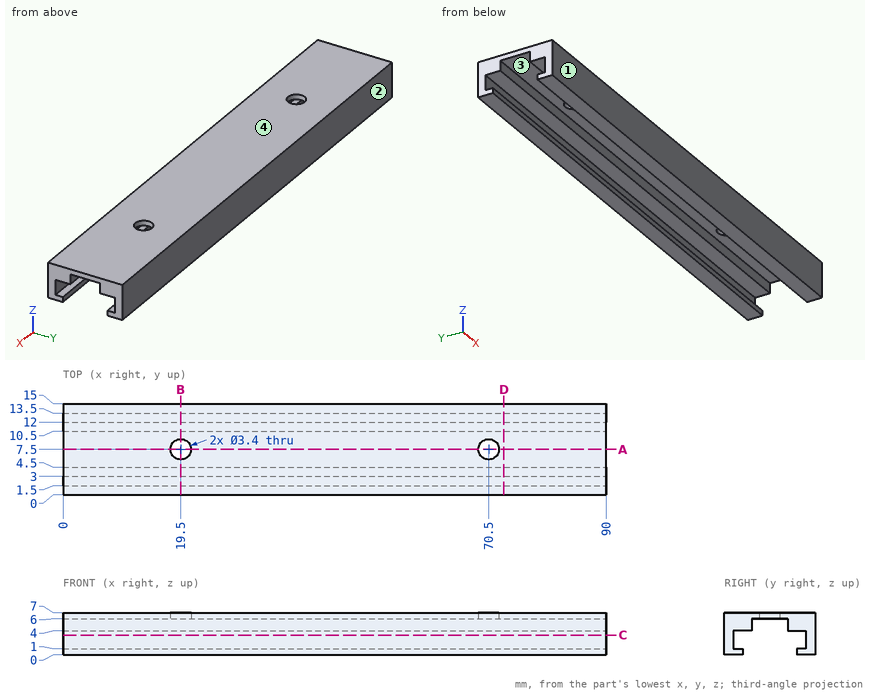
Could you check a few things on this drawing? It's one solid part, dimensions in mm from its lowest x, y, z. Coordinates: 2 decimals unless noted, no trailing zeros. Order: outer loops, then holes, each group sorted by start corner. A loop starts at its lowest first (then second) coordinate and runs counter-clockwise, first axis right, second up. Notation, with made-up numbers: (-39, -7.5) - (-13, -7.5) arc R15 ccw to (-13, 17.5) - close; hole circle Ø1 at (83.25, 55). An arc over 180 degrees is marked (long way). Answer as a JSON object with one key per item and string values. Group by question number.
Q1. Will this pin go through, and if not, where does the flat tip stop? P1, Ø6.5, axis at x = 47.5, y = 7, coming from the -Z side.
Q2. Imagine slicing it at A-A (y = 7.5). Please give me the cut outline in (x, z), and give its area (3 significant figures).
Q3. Imagine slicing it at B-B (x = 19.5). Please give me the cut outline in (y, z), and give its area (3 significant figures).
Q4. Imagine slicing it at C-C (z = 3.25). Please give me the cut outline in (x, y).
Q5. Imagine slicing it at D-D (x = 73). Please give me the cut outline in (y, z), and give its area (3 significant figures).
Q6. We'd pull the mould along Y, two halves only. Please class the marked faces 1, 2, 3 and 4: +Y half, -Y half, draft (parallel to the pull), parting line (faces both ways), or undercut.
Q7. I need wall thicknesses on line 1 (X direction, y = 7.5, z = 6.6); line 2 (Z direction, x = 21, y = 2); line 3 (Y direction, x = 19.5, z = 6.25). Which ranges of each line are inside material? Lowest first, please. Write a range as from..to.
Determined:
{
 "1": {"P1": "stops at z = 4"},
 "2": {"outline": "(0, 6) - (17.8, 6) - (17.8, 7) - (0, 7) - close; (21.2, 6) - (68.8, 6) - (68.8, 7) - (21.2, 7) - close; (72.2, 6) - (90, 6) - (90, 7) - (72.2, 7) - close", "area": "83.2 mm2"},
 "3": {"outline": "(0, 0) - (3, 0) - (3, 1) - (1.5, 1) - (1.5, 4) - (4.5, 4) - (4.5, 6) - (5.8, 6) - (5.8, 7) - (0, 7) - close; (9.2, 6) - (10.5, 6) - (10.5, 4) - (13.5, 4) - (13.5, 1) - (12, 1) - (12, 0) - (15, 0) - (15, 7) - (9.2, 7) - close", "area": "44.6 mm2"},
 "4": {"outline": "(0, 0) - (90, 0) - (90, 1.5) - (0, 1.5) - close; (0, 13.5) - (90, 13.5) - (90, 15) - (0, 15) - close"},
 "5": {"outline": "(0, 0) - (3, 0) - (3, 1) - (1.5, 1) - (1.5, 4) - (4.5, 4) - (4.5, 6) - (10.5, 6) - (10.5, 4) - (13.5, 4) - (13.5, 1) - (12, 1) - (12, 0) - (15, 0) - (15, 7) - (0, 7) - close", "area": "48.0 mm2"},
 "6": {"face 1": "-Y half", "face 2": "+Y half", "face 3": "undercut", "face 4": "draft"},
 "7": {"line 1": "x = 0..17.8, 21.2..68.8, 72.2..90", "line 2": "z = 0..1, 4..7", "line 3": "y = 0..5.8, 9.2..15"}
}
